from build123d import *

# Parameters (mm, degrees)
F1_DEPTH = 63.5
F0_W     = 25.3930282362
F0_H     = 19.05
F2_DEPTH = 50.8
F3_DEPTH = 7.9375


with BuildPart() as f1:
    # F0 (on Front) → F1 (new body, symmetric)
    with BuildSketch(Plane.XZ):
        Polygon((-41.275, 9.525), (-41.275, -9.525), (41.275, -9.525), (41.275, 9.525), (22.225, 9.525), align=None)
    extrude(amount=F1_DEPTH, both=True)

    # F0 (on Front) → F2 (join)
    with BuildSketch(Plane.XZ):
        with Locations((85.1897055026, 52.4002)):
            Rectangle(F0_W, F0_H)
        with BuildLine():
            Line((22.225, 9.525), (41.275, 9.525))
            Line((41.275, 9.525), (41.275, 27.0002))
            ThreePointArc((41.275, 27.0002), (45.9246798487, 38.2255201513), (57.15, 42.8752))
            Line((57.15, 42.8752), (72.4931913845, 42.8752))
            Line((72.4931913845, 42.8752), (72.4931913845, 61.9252))
            Line((72.4931913845, 61.9252), (57.15, 61.9252))
            add(Edge.make_bspline(
                [(54.1357817201, 61.7948851281), (55.1598986423, 61.8639699544), (56.1652679987, 61.9077817435), (57.15, 61.9252)],
                knots=[108.4182059101, 108.4182059101, 108.4182059101, 108.4182059101, 111.5045361635, 111.5045361635, 111.5045361635, 111.5045361635], degree=3))
            ThreePointArc((54.1357817201, 61.7948851281), (31.4106604744, 50.6061743664), (22.225, 27.0002))
            Line((22.225, 27.0002), (22.225, 9.525))
        make_face()
    extrude(amount=F2_DEPTH)

    # F0 (on Front) → F3 (join, symmetric)
    with BuildSketch(Plane.XZ):
        with BuildLine():
            add(Edge.make_bspline(
                [(-41.275, 9.525), (-40.9503712961, 25.7539404931), (18.1600726333, 59.3680376075), (54.1357817201, 61.7948851281)],
                knots=[0, 0, 0, 0, 108.4182059101, 108.4182059101, 108.4182059101, 108.4182059101], degree=3))
            Line((-41.275, 9.525), (22.225, 9.525))
            Line((22.225, 9.525), (22.225, 27.0002))
            ThreePointArc((22.225, 27.0002), (31.4106604744, 50.6061743664), (54.1357817201, 61.7948851281))
        make_face()
    extrude(amount=F3_DEPTH, both=True)


solid = f1.part
Geometry check sheet. Reference: the model listing, model coordinates, mm. A direction names the side the tool comes from. Give positions to 0.01 mm unless a question says otherwise; leave off trailing zeros. Order: outer loops, then holes, each group sorted by start corner. A loop starts at its lowest first (then second) coordinate and runs counter-clockwise, first axis right, second up. Notation, with made-up numbers: (26.5, -17.5) - (46.5, -17.5) arc R12 cw to (46.5, 2.5) - close; hole circle Ø1 at (-38, 7). An arc over 180 degrees is marked (long way). Use one line per item in the form item = value.
1) Material ranges on probe 1 along X at (y, z) = (-16, 28); probe 2 along Z at (x, y) = (19, -32) (3 decimals); probe 3 along Y at (x, z) = (39, 42.5), recorded low to high. Write a range as from..to.
Working result:
probe_1 = 22.24..41.31
probe_2 = -9.525..9.525
probe_3 = -50.8..0
2) Depth check by flat-ended pin: pin 1 Ø2 at (y, z) = (-38.5, 32) entering from -X; pin 2 Ø5 at (x, y) = (-3, -35) entering from +Z (3 decimals); pin 3 Ø14 at (y, z) = (-30, 19) entering from -X (3 decimals); pin 4 Ø3 at (x, z) = (20, 10.5) entering from -Y. Enter the tip coordinate at first touch or a pass-through.
Working result:
pin_1 = 22.45
pin_2 = 9.525
pin_3 = 22.225
pin_4 = -63.5
3) Sectioned sample at B-B (x = 64). Record the boundary of the cut face in (y, z), and give its area (3 significant figures).
Working result:
outline = (-50.8, 42.88) - (0, 42.88) - (0, 61.93) - (-50.8, 61.93) - close
area = 968 mm^2
4) Sectioned sample at A-A (y = 13). Record the boundary of the cut face in (x, z) (3 decimals).
Working result:
outline = (-41.275, -9.525) - (41.275, -9.525) - (41.275, 9.525) - (-41.275, 9.525) - close
5) Draft check along Z on faces 4 (the face through (-1, -1, -9.525)), 5 (the face through (41.275, -1, 4)), 6 (the face through (31.17, 3.91, 50.34)). Enter one of: released by +Z, released by -Z, zero draft, split by the parting line, or undercut.
Working result:
face_4 = released by -Z
face_5 = zero draft
face_6 = undercut
6) Access from +Z, -Z, +X, -X, +Y, -Y to the whole of each face (thin tool, end or side, straight path). Record for faces 1 (the face through (-4, 7.938, 30)), 2 (the face through (51, 0, 42)), 3 (the face through (-4, -7.938, 30)).
Working result:
face_1 = +Z, +X, -X, +Y
face_2 = +X, +Y
face_3 = +Z, -X, -Y
